Read the model definition and answer for the solid it produces. Units are mm, in the model's axes. A direction names the side the tool comes from. Coordinates: 2 decimals unless noted, no trailing zeros. Loops run counter-clockwise (first coordinate to the right, second up) from the corner with the lowest first, then second, coordinate; pieces in that order, holes last. Notation, with made-up numbers: (-24.5, 50.5) - (-12.5, 50.5) arc R27 ccw to (-12.5, 70.5) - close; hole circle Ø7 at (36.25, 89.25). An arc over 180 degrees is marked (long way). Use CSV: the item, a comma, the result in double quotes.
```python
from build123d import *

# Parameters (mm, degrees)
F4_W     = 110
F4_H     = 56
F4_W_2   = 103.5
F4_H_2   = 49.5
F5_DEPTH = 2
F6_DEPTH = 4.3
F7_R     = 3
F8_R     = 1


with BuildPart() as f5:
    # F4 (on Top) → F5 (new body)
    with BuildSketch(Plane.XY):
        Rectangle(F4_W, F4_H)
        Rectangle(F4_W_2, F4_H_2, mode=Mode.SUBTRACT)
        Rectangle(F4_W_2, F4_H_2)
    extrude(amount=-F5_DEPTH)

    # F4 (on Top) → F6 (join)
    with BuildSketch(Plane.XY):
        Rectangle(F4_W, F4_H)
        Rectangle(F4_W_2, F4_H_2, mode=Mode.SUBTRACT)
    extrude(amount=F6_DEPTH)

    # F7
    f7_edges = [f5.edges().sort_by_distance(p)[0] for p in [
        (-55, -28, 1.15),
        (55, -28, 1.15),
        (55, 28, 1.15),
        (-55, 28, 1.15),
    ]]
    fillet(f7_edges, radius=F7_R)

    # F8
    f8_edges = [f5.edges().sort_by_distance(p)[0] for p in [
        (0, 28, -2),
        (54.12132, 27.12132, -2),
        (-54.12132, 27.12132, -2),
        (55, 0, -2),
        (-55, 0, -2),
        (54.12132, -27.12132, -2),
        (-54.12132, -27.12132, -2),
        (0, -28, -2),
    ]]
    fillet(f8_edges, radius=F8_R)


solid = f5.part
```
Q1. For a pull along X with two mould halves and no side action, classify faces 3 (the face through (-1, -28, 2)), 4 (the face through (-1, -24.75, 2)), 5 (the face through (-55, 0, 2)) as +X half, -X half, draft (parallel to the pull), parting line (faces both ways), or undercut.
Reported:
face 3,"draft"
face 4,"undercut"
face 5,"-X half"
Q2. The part is cut by section C-C on y = 13.5. Determine the outline of the cut face in (x, z).
Reported:
outline,"(-55, -1) arc R1 ccw to (-54, -2) - (54, -2) arc R1 ccw to (55, -1) - (55, 4.3) - (51.75, 4.3) - (51.75, 0) - (-51.75, 0) - (-51.75, 4.3) - (-55, 4.3) - close"
Q3. A tool of negligible diameter and unlimited length cuts with its end or side. For faces 1 (the face through (-54.14, 27.1, 1.61)), 2 (the face through (-1, 0, 0)), from which of +Z, -Z, +X, -X, +Y, -Y can it reach the whole face along a straight path? Write none if from no direction.
Reported:
face 1,"+Z, -Z, -X, +Y"
face 2,"+Z"
Q4. Find the intervals of material crossed by probe 1 along Y at (x, z) = (-23, 1.25); probe 2 along X at (y, z) = (18.5, 1); probe 3 along Z at (x, y) = (-30, 19.5), in increasing order. Write a range as [from, to].
Reported:
probe 1,"y = [-28, -24.75], [24.75, 28]"
probe 2,"x = [-55, -51.75], [51.75, 55]"
probe 3,"z = [-2, 0]"
Q5. The part is cut by section B-B on x = 42.5. Determine the outline of the cut face in (y, z), and give its area (3 significant figures).
Reported:
outline,"(-28, -1) arc R1 ccw to (-27, -2) - (27, -2) arc R1 ccw to (28, -1) - (28, 4.3) - (24.75, 4.3) - (24.75, 0) - (-24.75, 0) - (-24.75, 4.3) - (-28, 4.3) - close"
area,"140 mm²"
Q6. The part is cut by section A-A on z = 3.25. Determine the outline of the cut face in (x, y), and give its area (3 significant figures).
Reported:
outline,"(-55, -25) arc R3 ccw to (-52, -28) - (52, -28) arc R3 ccw to (55, -25) - (55, 25) arc R3 ccw to (52, 28) - (-52, 28) arc R3 ccw to (-55, 25) - close; hole (-51.75, -24.75) - (51.75, -24.75) - (51.75, 24.75) - (-51.75, 24.75) - close"
area,"1,030 mm²"
Q7. Given P1, Ø3, axis at x = 2, y = -19.5, coming from the +Z side, flat-ended and moving along its own axis, determine where the tip first touches the part or whether it passes through.
Reported:
P1,"stops at z = 0"
